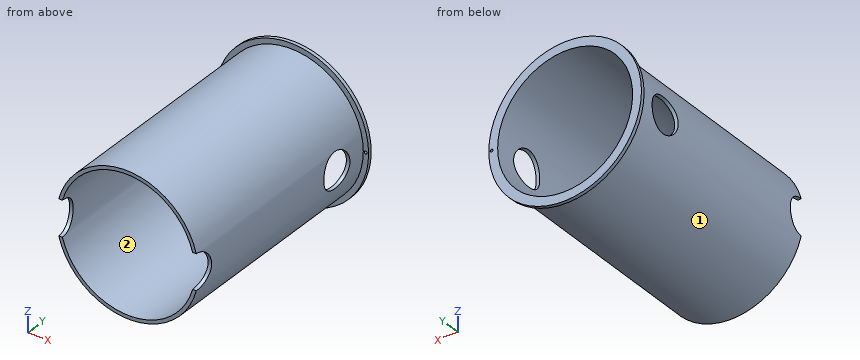
Autodesk Inventor part; units mm, degrees
ref_plane "YZ Plane" through (0, 0, 0) normal (1, 0, 0) x (0, 1, 0)
ref_plane "XZ Plane" through (0, 0, 0) normal (0, 1, 0) x (-1, 0, 0)
ref_plane "XY Plane" through (0, 0, 0) normal (0, 0, 1) x (1, 0, 0)
sketch "Эскиз1" plane through (0, 0, 0) normal (0, 0, 1) x (1, 0, 0)
  line L0 (0, 0) -> (190, 0)
  line L1 (190, 0) -> (190, 640)
  line L2 (190, 640) -> (215, 640)
  line L3 (215, 640) -> (215, 630)
  line L4 (215, 630) -> (200, 630)
  line L5 (200, 630) -> (200, 0)
  line L6 (200, 0) -> (190, 0)
  line L7 (0, -128) -> (0, 768)
  dimension "d0" = 190
  dimension "d1" = 640
  dimension "d2" = 25
  dimension "d3" = 10
revolve "Вращение1" add sketch "Эскиз1" angle 360 about axis through (0, -10, 0) along (0, 1, 0)
sketch "Эскиз2" plane through (0, 640, 0) normal (0, 1, 0) x (1, 0, 0)
  circle A0 centre (207, 0) radius 4
  circle A1 centre (0, 0) radius 190
  line L0 (190, 0) -> (207, 0)
  dimension "d6" = 8
  dimension "d19" = 17
extrude "Выдавливание1" cut sketch "Эскиз2" against normal through all contours A0
sketch "Эскиз3" plane through (0, 0, 0) normal (1, 0, 0) x (0, 1, 0)
  line L0 (630, 215) -> (630, -215)
  line L1 (630, 200) -> (630, -200)
  line L2 (630, 0) -> (529, 0)
  circle A0 centre (529, 0) radius 50
  line L3 (0, 0) -> (0, 0)
  circle A1 centre (0, 0) radius 50
  dimension "d11" = 101
  dimension "d12" = 100
  dimension "d17" = 0
  dimension "d18" = 100
extrude "Выдавливание2" cut sketch "Эскиз3" along normal through all both and the other way through all
properties part number "Втулка" material "Сталь, легированная"
Source: CAD feature listing. Evaluate the final solid. Frame: model axes, mm. Face numbers are marked on the shaded views. Coordinates: 2 decimals unless noted, no trailing zeros. Write each loop counter-clockwise with the first axis right and the second up, starting at its lowest first coordinate (ties: lowest second). Pieces come first, ordered by that corner, then holes. Notation, with made-up numbers: (84, 21.5) -> (124, 21.5) arc R22 cw to (124, 50.5) -> close; hole circle Ø9 at (29.25, 73.25). An arc over 180 degrees is marked (long way). Return JSON: item names as keys, results as strings. Group by question number.
1) Mould query, pull axis Z, two halves, no side actions, for the marked faces 1 and 2. Classes: +Z half, -Z half, draft (parallel to the pull), parting line (faces both ways), or undercut.
2) Section query A-A, the plane y = 529. Return loops of the section in (x, z).
3) Contact query for flat-ended pins moving along their axis: P1, Ø8, axis at x = 158, y = 526, coming from the -Z side; P2, Ø4, axis at x = -109, y = 422.5, coming from the -Z side; P3, Ø2, axis at x = -12, y = 334.5, coming from the +Z side. Output: stop coordinate, or through.
4) Section query B-B, the plane x = 0. Return loops of the section in (y, z).
5) Ray query, line 1 along X through (y, z) = (346, 0); line 2 along Y through (x, z) = (193, 0); line 3 along X through (y, z) = (385, -9.5). Return the intervals inside material, ascending.
6) Section query D-D, the plane y = 263.5. Return loops of the section in (x, z), plus the area to 3 significant figures.
7) Section query C-C, the plane z = 35. Return loops of the section in (x, y), plus the area to 3 significant figures.
From the geometry:
{
 "1": {"face 1": "parting line", "face 2": "undercut"},
 "2": {"outline": "(-193.65, -50) arc R200 ccw to (193.65, -50) -> (183.3, -50) arc R190 cw to (-183.3, -50) -> close; (-193.65, 50) -> (-183.3, 50) arc R190 cw to (183.3, 50) -> (193.65, 50) arc R200 ccw to start"},
 "3": {"P1": "z = -127.61", "P2": "z = -168.97", "P3": "z = 199.7"},
 "4": {"outline": "(0, -200) -> (630, -200) -> (630, -215) -> (640, -215) -> (640, -190) -> (0, -190) -> close; (0, 190) -> (640, 190) -> (640, 215) -> (630, 215) -> (630, 200) -> (0, 200) -> close"},
 "5": {"line 1": "-200 to -190, 190 to 200", "line 2": "50 to 479, 579 to 640", "line 3": "-199.77 to -189.76, 189.76 to 199.77"},
 "6": {"outline": "circle Ø400 at (0, 0); hole circle Ø380 at (0, 0)", "area": "12,300 mm²"},
 "7": {"outline": "(-212.13, 630) -> (-196.91, 630) -> (-196.91, 564.71) -> (-186.75, 564.71) -> (-186.75, 640) -> (-212.13, 640) -> close; (-196.91, 35.71) -> (-186.75, 35.71) -> (-186.75, 493.29) -> (-196.91, 493.29) -> close; (186.75, 35.71) -> (196.91, 35.71) -> (196.91, 493.29) -> (186.75, 493.29) -> close; (186.75, 564.71) -> (196.91, 564.71) -> (196.91, 630) -> (212.13, 630) -> (212.13, 640) -> (186.75, 640) -> close", "area": "11,100 mm²"}
}
